from build123d import *

# Parameters (mm, degrees)
SKETCH_1_R          = 5
EXTRUDE_1_DEPTH     = 10
SKETCH_1_3_W        = 10
SKETCH_1_3_H        = 5
EXTRUDE_2_DEPTH     = 15
SKETCH_1_4_W        = 5
SKETCH_1_4_H        = 20
EXTRUDE_3_DEPTH     = 20
CUT_EXTRUDE_1_DEPTH = 20
SCALE_1_SCALE       = 0.2


with BuildPart() as part:
    # Sketch 1 → Extrude 1 (new body)
    with BuildSketch(Plane(origin=(0, 0, 0), x_dir=(1, 0, 0), z_dir=(0, 1, 0))):
        Polygon((10, 15), (5, 15), (5, 10), (-5, 10), (-10, 10), (-10, -10), (10, -10), align=None)
        Circle(SKETCH_1_R, mode=Mode.SUBTRACT)
    extrude(amount=EXTRUDE_1_DEPTH)

    # Sketch 1_3 → Extrude 2 (add)
    with BuildSketch(Plane(origin=(0, 0, 0), x_dir=(1, 0, 0), z_dir=(0, 1, 0))):
        with Locations((0, 12.5)):
            Rectangle(SKETCH_1_3_W, SKETCH_1_3_H)
    extrude(amount=EXTRUDE_2_DEPTH)

    # Sketch 1_4 → Extrude 3 (add)
    with BuildSketch(Plane(origin=(0, 0, 0), x_dir=(1, 0, 0), z_dir=(0, 1, 0))):
        Polygon((-5, 15), (-15, 15), (-15, 10), (-10, 10), (-5, 10), align=None)
        with Locations((-12.5, 0)):
            Rectangle(SKETCH_1_4_W, SKETCH_1_4_H)
    extrude(amount=EXTRUDE_3_DEPTH)

    # Sketch 2 → Cut-Extrude 1 (cut)
    with BuildSketch(Plane(origin=(-10, 0, 0), x_dir=(0, 0, -1), z_dir=(1, 0, 0))):
        Polygon((-10, 10), (10, 20), (-10, 20), align=None)
    extrude(amount=-CUT_EXTRUDE_1_DEPTH, mode=Mode.SUBTRACT)


with BuildPart() as part_1:
    # Scale 1: scaled about (-4.00247113, 6.644426123, -3.971444222)
    add(part.part.scale(SCALE_1_SCALE).moved(Location((-3.201976904, 5.315540898, -3.177155378))))


solid = part_1.part
Geometry check sheet. Reference: the model listing, model coordinates, mm. A direction names the side the tool comes from. Give positions to 0.01 mm unless a question says otherwise; leave off trailing zeros. Order: outer loops, then holes, each group sorted by start corner. A loop starts at its lowest first (then second) coordinate and runs counter-clockwise, first axis right, second up. Notation, with made-up numbers: (43, 80) - (53, 80) arc R20 ccw to (53, 105) - close; hole circle Ø3 at (68.25, 47). An arc over 180 degrees is marked (long way). Use one line per item in the form item = value.
1) Sectioned sample at C-C (z = -5.5). Record the boundary of the cut face in (x, y), and give its area (3 significant figures).
Working result:
outline = (-6.2, 5.32) - (-1.2, 5.32) - (-1.2, 7.32) - (-2.2, 7.32) - (-2.2, 8.32) - (-4.2, 8.32) - (-4.2, 9.32) - (-6.2, 9.32) - close
area = 16.0 mm^2
2) Sectioned sample at A-A (z = -3.7). Record the boundary of the cut face in (x, y), and give its area (3 significant figures).
Working result:
outline = (-6.2, 5.32) - (-4.05, 5.32) - (-4.05, 7.32) - (-5.2, 7.32) - (-5.2, 8.58) - (-6.2, 8.58) - close; (-2.35, 5.32) - (-1.2, 5.32) - (-1.2, 7.32) - (-2.35, 7.32) - close
area = 7.85 mm^2
3) Sectioned sample at B-B (x = -3.9). Record the boundary of the cut face in (y, z).
Working result:
outline = (5.32, -6.18) - (8.32, -6.18) - (8.32, -5.18) - (7.32, -5.18) - (7.32, -3.89) - (5.32, -3.89) - close; (5.32, -2.46) - (7.32, -2.46) - (7.32, -1.18) - (5.32, -1.18) - close
4) Access from +Z, -Z, +X, -X, +Y, -Y to the whole of each face (thin tool, end or side, straight path). Record for faces 1 (the face through (-4.3, 5.316, -3.7)), 2 (the face through (-4, 8, -5.177)), 3 (the face through (-2.202, 8, -6)).
Working result:
face_1 = +Z, -Z, +X, -X, -Y
face_2 = +Z, +X, +Y
face_3 = +Z, -Z, +X, +Y
5) Draft check along X on faces 4 (the face through (-5.202, 8, -4)), 5 (the face through (-2.74, 6.3, -2.29)), 6 (the face through (-4, 7, -6.177)). Enter one of: released by +X, released by -X, zero draft, split by the parting line, or undercut.
Working result:
face_4 = released by +X
face_5 = undercut
face_6 = zero draft
6) Sectioned sample at D-D (x = -5.45). Record the boundary of the cut face in (y, z).
Working result:
outline = (5.32, -6.18) - (9.32, -6.18) - (9.32, -5.18) - (7.32, -1.18) - (5.32, -1.18) - close
7) Material ranges on probe 1 along Z at (x, y) = (-3.2, 5.7); probe 2 along X at (y, z) = (7.35, -1.6); probe 3 along Y at (x, z) = (-2.6, -1.85), recorded low to high. Write a range as from..to.
Working result:
probe_1 = -6.18..-4.18, -2.18..-1.18
probe_2 = -6.2..-5.2
probe_3 = 5.32..7.32
8) Depth check by flat-ended pin: pin 1 Ø1.1 at (x, z) = (-3, -5.5) entering from +Y; pin 2 Ø1 at (x, y) = (-3, 8.5) entering from +Z; pin 3 Ø1.2 at (x, z) = (-3.2, -3.18) entering from +Y; pin 4 Ø0.5 at (y, z) = (8.5, -5.5) entering from +X. Enter the tip coordinate at first touch or a pass-through.
Working result:
pin_1 = 8.32
pin_2 = -5.18
pin_3 = through
pin_4 = -2.2
